Geometry: see drawing. Coordinates: mm, zero at the bounding-box minimum. A direction names the side the tool comes from. Round coordinates to 2 decimals unless told otherwise and drop trailing zeros. Loops run counter-clockwise (first coordinate to the right, second up) from the corner with the lowest first, then second, coordinate; pieces in that order, holes last.
(1) Section B-B, the plane x = 16.51. Return the cut outline in (y, z) (3 decimals).
(2) Section C-C, the plane y = 5.08. Return the cut outline in (x, z), plus the area to 3 significant figures.
(3) Section D-D, the plane y = 3.5. Return the cut outline in (x, z).
(4) Mould query, pull axis X, two halves, no side actions, for the marked faces 1, 2 and 3. Classes: pulls with the +X half, pulls with the -X half, needs draft (parallel to the pull), parting line crosses it, or undercut.
(5) First-contact query: pin 1 Ø3.5 at (x, y) = (16.51, 5.08) entering from -Z; pin 2 Ø5 at (x, y) = (7.5, 3) entering from +Z; pin 3 Ø1 at (x, z) = (7.5, 3.5) entering from -Y. Flat tips, straight axial feed; report the tip coordinate or a pass-through.
(6) Set-up query: the marked faces 4, 5 and 6. Return all of +Z, -Z, +X, -X, +Y, -Y with unobstructed straight access to the full face (end or side cutting, diameter ignored); none if empty.
(7) Material intervals for probe 1 along Y at (x, z) = (16.51, 2.4) (3 decimals); probe 2 along X at (y, z) = (3, 4); probe 3 along Y at (x, z) = (16.51, 0.45), sorted ascending.
(8) Section A-A, the plane z = 4.4. Return the cut outline in (x, y) (3 decimals).
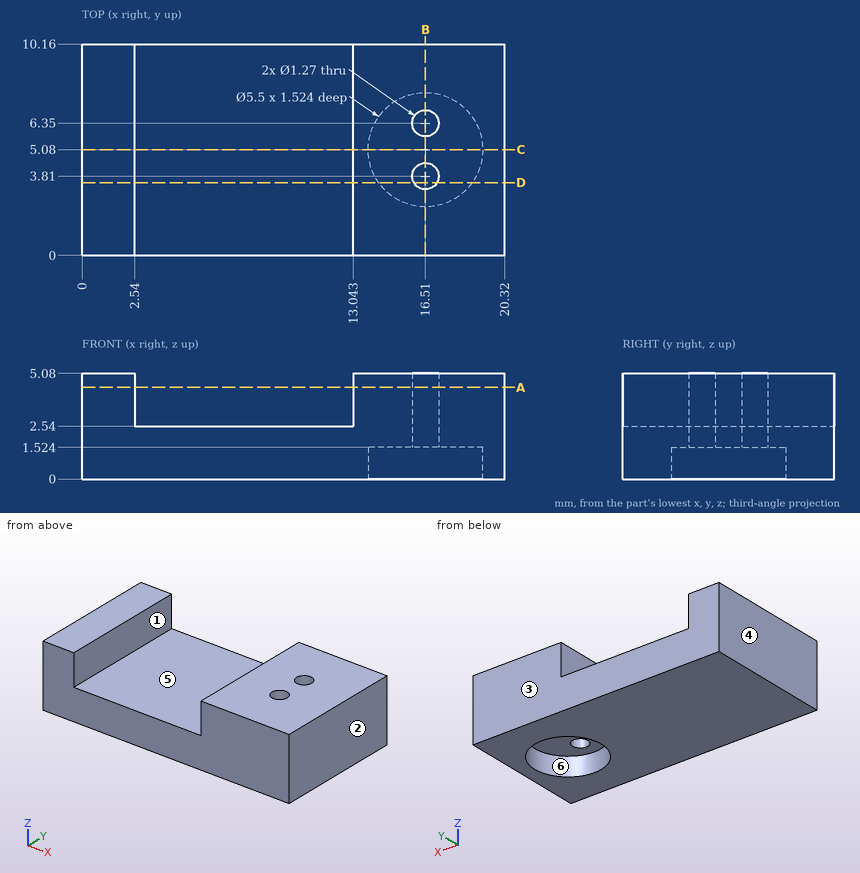
Output values:
1. outline: (0, 0) - (2.33, 0) - (2.33, 1.524) - (3.175, 1.524) - (3.175, 5.08) - (0, 5.08) - close; (4.445, 1.524) - (5.715, 1.524) - (5.715, 5.08) - (4.445, 5.08) - close; (6.985, 1.524) - (7.83, 1.524) - (7.83, 0) - (10.16, 0) - (10.16, 5.08) - (6.985, 5.08) - close
2. outline: (0, 0) - (13.76, 0) - (13.76, 1.52) - (19.26, 1.52) - (19.26, 0) - (20.32, 0) - (20.32, 5.08) - (13.04, 5.08) - (13.04, 2.54) - (2.54, 2.54) - (2.54, 5.08) - (0, 5.08) - close
2. area: 68.2 mm2
3. outline: (0, 0) - (14.26, 0) - (14.26, 1.52) - (15.96, 1.52) - (15.96, 5.08) - (13.04, 5.08) - (13.04, 2.54) - (2.54, 2.54) - (2.54, 5.08) - (0, 5.08) - close; (17.06, 1.52) - (18.76, 1.52) - (18.76, 0) - (20.32, 0) - (20.32, 5.08) - (17.06, 5.08) - close
4. face 1: undercut
4. face 2: pulls with the +X half
4. face 3: needs draft
5. pin 1: stops at z = 1.52
5. pin 2: stops at z = 2.54
5. pin 3: passes through
6. face 4: +Z, -Z, -X, +Y, -Y
6. face 5: +Z, +Y, -Y
6. face 6: -Z
7. probe 1: y = 0 to 3.175, 4.445 to 5.715, 6.985 to 10.16
7. probe 2: x = 0 to 2.54, 13.04 to 20.32
7. probe 3: y = 0 to 2.33, 7.83 to 10.16
8. outline: (0, 0) - (2.54, 0) - (2.54, 10.16) - (0, 10.16) - close; (13.043, 0) - (20.32, 0) - (20.32, 10.16) - (13.043, 10.16) - close; hole circle Ø1.27 at (16.51, 3.81); hole circle Ø1.27 at (16.51, 6.35)
